Could you check a few things on this model? Use its own coordinates, in mm. Face numbers are marked on the shaded views. A direction names the side the tool comes from. Give positions to 0.01 mm unless a question says otherwise; leave off trailing zeros. Loops run counter-clockwise (first coordinate to the right, second up) from the corner with the lowest first, then second, coordinate; pieces in that order, holes last.
1. Imagine slicing it at C-C (y = 0). List the corners of the cut face in (x, z) for me (3 decimals), plus the area to 3 significant figures.
2. Imagine slicing it at D-D (x = 8.5). List the corners of the cut face in (y, z) for me.
3. Thinking about a two-plate mould opening in Y: for the marked faces 3, 4 and 5, which applies, +Y half, -Y half, draft (parallel to the pull), parting line (faces both ways), or undercut?
4. For P1, Ø10.5, axis at x = 0, y = 0, coming from the +Z side; P2, Ø6, axis at y = 16, z = 22.5, coming from the -X side; P3, Ø1, axis at y = 20, z = 14.5, coming from the +X side, each with a flat end and sliding along its axis, tell me the tip position at first contact or that it passes through.
5. Imagine slicing it at B-B (z = 32.5). List the corners of the cut face in (x, y) for me (3 decimals), plus the area to 3 significant figures.
6. I need wall thicknesses on line 1 along Y through (x, z) = (-10.5, 35); line 2 along X through (y, z) = (10.5, 38); line 3 along Y through (x, z) = (0, 17) (3 decimals). Which ranges of each line are inside material? Lowest first, please.
7. Imagine slicing it at A-A (x = -17). List the corners of the cut face in (y, z) for me, plus the area to 4 significant figures.
8. For the marked faces 1 and 2, which set-ups out of +Z, -Z, +X, -X, +Y, -Y let a thin tool reach every point of the face, with its end or its side?
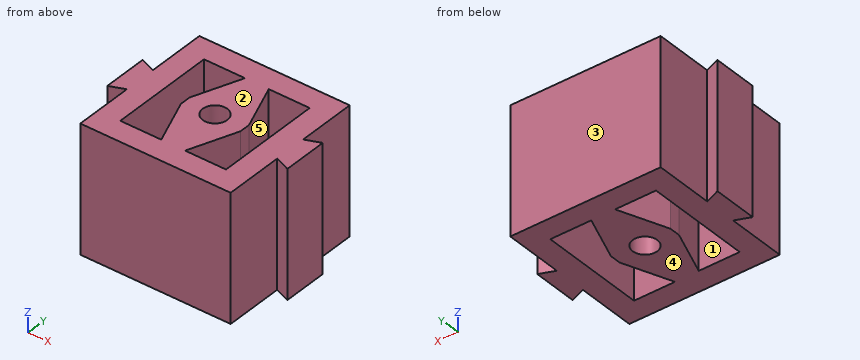
```python
from build123d import *

# Parameters (mm, degrees)
SKETCH1_W           = 50.5
SKETCH1_H           = 50.5
BOSS_EXTRUDE1_DEPTH = 42.5
SKETCH2_R           = 4.125
CUT_EXTRUDE1_DEPTH  = 46.2
CUT_EXTRUDE2_DEPTH  = 76


with BuildPart() as part:
    # Sketch1 → Boss-Extrude1 (new body)
    with BuildSketch(Plane.XY):
        Rectangle(SKETCH1_W, SKETCH1_H)
        Polygon((-25.25, -5.5), (-25.25, 5.5), (-30.25, 7.5), (-30.25, -7.5), align=None)
        Polygon((30.25, 7.5), (25.25, 5.5), (25.25, -5.5), (30.25, -7.5), align=None)
    extrude(amount=BOSS_EXTRUDE1_DEPTH)

    # Sketch2 → Cut-Extrude1 (cut)
    with BuildSketch(Plane.XY.offset(42.5)):
        Circle(SKETCH2_R)
    extrude(amount=-CUT_EXTRUDE1_DEPTH, mode=Mode.SUBTRACT)

    # Sketch4 → Cut-Extrude2 (cut)
    with BuildSketch(Plane.XY.offset(42.5)):
        Polygon((-17.75, -17.75), (-17.75, 17.75), (-4, 17.75), (-10, 1.820899919), (-10, -1.820899919), (-4, -17.75), align=None)
        Polygon((10, -1.820899919), (4, -17.75), (17.75, -17.75), (17.75, 17.75), (4, 17.75), (10, 1.820899919), align=None)
    extrude(amount=-CUT_EXTRUDE2_DEPTH, mode=Mode.SUBTRACT)


solid = part.part
```
Derived:
1. outline: (-30.25, 0) - (-17.75, 0) - (-17.75, 42.5) - (-30.25, 42.5) - close; (-10, 0) - (-4.125, 0) - (-4.125, 42.5) - (-10, 42.5) - close; (4.125, 0) - (10, 0) - (10, 42.5) - (4.125, 42.5) - close; (17.75, 0) - (30.25, 0) - (30.25, 42.5) - (17.75, 42.5) - close
1. area: 1,560 mm2
2. outline: (-25.25, 0) - (-17.75, 0) - (-17.75, 42.5) - (-25.25, 42.5) - close; (-5.8, 0) - (5.8, 0) - (5.8, 42.5) - (-5.8, 42.5) - close; (17.75, 0) - (25.25, 0) - (25.25, 42.5) - (17.75, 42.5) - close
3. face 3: +Y half
3. face 4: draft
3. face 5: undercut
4. P1: stops at z = 42.5
4. P2: stops at x = -25.25
4. P3: stops at x = 25.25
5. outline: (-30.25, -7.5) - (-25.25, -5.5) - (-25.25, -25.25) - (25.25, -25.25) - (25.25, -5.5) - (30.25, -7.5) - (30.25, 7.5) - (25.25, 5.5) - (25.25, 25.25) - (-25.25, 25.25) - (-25.25, 5.5) - (-30.25, 7.5) - close; hole (-17.75, -17.75) - (-4, -17.75) - (-10, -1.821) - (-10, 1.821) - (-4, 17.75) - (-17.75, 17.75) - close; hole circle Ø8.25 at (0, 0); hole (4, -17.75) - (17.75, -17.75) - (17.75, 17.75) - (4, 17.75) - (10, 1.821) - (10, -1.821) - close
5. area: 1,890 mm2
6. line 1: y = -25.25 to -17.75, 17.75 to 25.25
6. line 2: x = -25.25 to -17.75, -6.73 to 6.73, 17.75 to 25.25
6. line 3: y = -25.25 to -4.125, 4.125 to 25.25
7. outline: (-25.25, 0) - (-17.75, 0) - (-17.75, 42.5) - (-25.25, 42.5) - close; (17.75, 0) - (25.25, 0) - (25.25, 42.5) - (17.75, 42.5) - close
7. area: 637.5 mm2
8. face 1: +Z, -Z
8. face 2: +Z, +X, -X, +Y, -Y
